```python
from build123d import *

# Parameters (mm, degrees)
F0_W     = 100
F0_H     = 95
F1_DEPTH = 10
F3_DEPTH = 10
F4_R     = 3


with BuildPart() as f1:
    # F0 (on Top) → F1 (new body, symmetric)
    with BuildSketch(Plane.XY):
        Rectangle(F0_W, F0_H)
    extrude(amount=F1_DEPTH, both=True)

    # F2 (on face) → F3 (cut)
    with BuildSketch(Plane.XY.offset(10)):
        with BuildLine():
            Line((18.764, 40.500201), (-18.764, 40.500201))
            ThreePointArc((-18.764, 40.500201), (-22.764, 39.428405), (-25.692203, 36.500201))
            Line((-25.692203, 36.500201), (-44.456203, 4))
            ThreePointArc((-44.456203, 4), (-45.528, 0), (-44.456203, -4))
            Line((-44.456203, -4), (-25.692203, -36.500201))
            ThreePointArc((-25.692203, -36.500201), (-22.764, -39.428405), (-18.764, -40.500201))
            Line((-18.764, -40.500201), (18.764, -40.500201))
            ThreePointArc((18.764, -40.500201), (22.764, -39.428405), (25.692203, -36.500201))
            Line((25.692203, -36.500201), (44.456203, -4))
            ThreePointArc((44.456203, -4), (45.528, 0), (44.456203, 4))
            Line((44.456203, 4), (25.692203, 36.500201))
            ThreePointArc((25.692203, 36.500201), (22.764, 39.428405), (18.764, 40.500201))
        make_face()
    extrude(amount=-F3_DEPTH, mode=Mode.SUBTRACT)

    # F4
    f4_edges = [f1.edges().sort_by_distance(p)[0] for p in [
        (0, -47.5, 10),
        (0, 47.5, 10),
    ]]
    fillet(f4_edges, radius=F4_R)


solid = f1.part
```
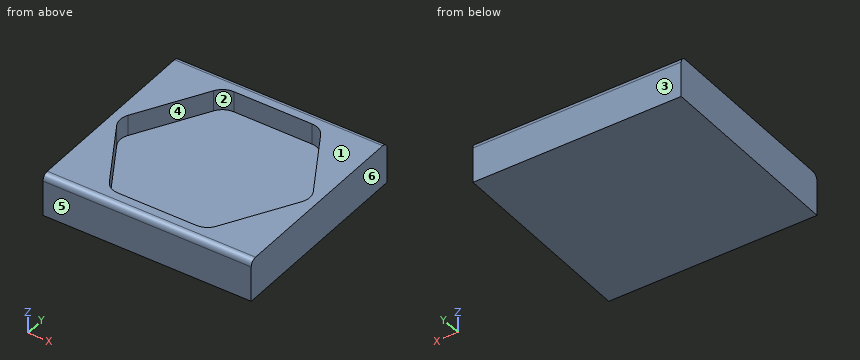
Geometry check sheet. Reference: the model listing, model coordinates, mm. Face numbers are marked on the shaded views. A direction names the side the tool comes from. Give positions to 0.01 mm unless a question says otherwise; leave off trailing zeros. Order: outer loops, then holes, each group sorted by start corner. A loop starts at its lowest first (then second) coordinate and runs counter-clockwise, first axis right, second up. Notation, with made-up numbers: (-26, 65.5) -> (26, 65.5) arc R11 cw to (26, 77.5) -> close; hole circle Ø6 at (21, 22). An arc over 180 degrees is marked (long way). Write each question's results on one line, items separated by ' | '. Start each with the question number.
(1) Sectioned sample at B-B (x = 4). Enter the section's corners in (y, z), plus the area to 3 significant figures.
(2) Scan lines: line 1 (Y direction, x = 1.5, z = 5); line 2 (Z direction, x = -11.5, y = -19.5); line 3 (Y direction, x = 21, z = 1). Record each from-to range of solid material in increasing order.
(3) Sectioned sample at A-A (z = 5.5). Enter the section's corners in (x, y).
(4) Gauge pin test, flat end, axial feed: P1, Ø5, axis at x = -39, y = -13, coming from the +Z side. Record the tip position at first contact, or that the pin passes through.
(5) Sectioned sample at D-D (y = 34.5). Enter the section's corners in (x, z), plus the area to 3 significant figures.
(6) Mould release check, pull along Y, two halves, no side actions. Record for the marked faces 3, 4, 5 and 6: pulls with the +Y half, pulls with the -Y half, needs draft (parallel to the pull), parting line crosses it, or undercut.
(7) Sectioned sample at C-C (y = 0). Enter the section's corners in (x, z), plus the area to 3 significant figures.
(8) Access from +Z, -Z, +X, -X, +Y, -Y to the whole of each face (thin tool, end or side, straight path). Record for the marked faces 1 and 2.
Answer below:
1) outline: (-47.5, -10) -> (47.5, -10) -> (47.5, 7) arc R3 ccw to (44.5, 10) -> (40.5, 10) -> (40.5, 0) -> (-40.5, 0) -> (-40.5, 10) -> (-44.5, 10) arc R3 ccw to (-47.5, 7) -> close | area: 1,090 mm2
2) line 1: -47.5 to -40.5, 40.5 to 47.5 | line 2: -10 to 0 | line 3: -47.5 to -40.18, 40.18 to 47.5
3) outline: (-50, -47.5) -> (50, -47.5) -> (50, 47.5) -> (-50, 47.5) -> close; hole (-44.46, -4) -> (-25.69, -36.5) arc R8 ccw to (-18.76, -40.5) -> (18.76, -40.5) arc R8 ccw to (25.69, -36.5) -> (44.46, -4) arc R8 ccw to (44.46, 4) -> (25.69, 36.5) arc R8 ccw to (18.76, 40.5) -> (-18.76, 40.5) arc R8 ccw to (-25.69, 36.5) -> (-44.46, 4) arc R8 ccw to start
4) P1: z = 10
5) outline: (-50, -10) -> (50, -10) -> (50, 10) -> (26.85, 10) -> (26.85, 0) -> (-26.85, 0) -> (-26.85, 10) -> (-50, 10) -> close | area: 1,460 mm2
6) face 3: pulls with the +Y half | face 4: undercut | face 5: pulls with the -Y half | face 6: needs draft
7) outline: (-50, -10) -> (50, -10) -> (50, 10) -> (45.53, 10) -> (45.53, 0) -> (-45.53, 0) -> (-45.53, 10) -> (-50, 10) -> close | area: 1,090 mm2
8) face 1: +Z, +X, -X, +Y, -Y | face 2: +Z
